from build123d import *

# Parameters (mm, degrees)
SKETCH1_W               = 37
SKETCH1_H               = 52
BOSS_EXTRUDE1_DEPTH     = 2
BOSS_EXTRUDE2_DEPTH     = 52
SKETCH3_W               = 10.2
SKETCH3_H               = 48.4
CUT_EXTRUDE1_DEPTH      = 11
CUT_EXTRUDE2_DEPTH      = 35.456494308
CUT_EXTRUDE2_DEPTH_BACK = 35.456494308


with BuildPart() as part:
    # Sketch1 → Boss-Extrude1 (new body)
    with BuildSketch(Plane.XY):
        Rectangle(SKETCH1_W, SKETCH1_H)
    extrude(amount=BOSS_EXTRUDE1_DEPTH)

    # Sketch2 → Boss-Extrude2 (add)
    with BuildSketch(Plane.XZ.offset(26)):
        with BuildLine():
            Line((-13.5, 13), (13.5, 13))
            ThreePointArc((13.5, 13), (17.035533906, 11.535533906), (18.5, 8))
            Line((18.5, 8), (18.5, 2))
            Line((18.5, 2), (-18.5, 2))
            Line((-18.5, 2), (-18.5, 8))
            ThreePointArc((-18.5, 8), (-17.035533906, 11.535533906), (-13.5, 13))
        make_face()
    extrude(amount=-BOSS_EXTRUDE2_DEPTH)

    # Sketch3 → Cut-Extrude1 (cut)
    with BuildSketch(Plane.XY.offset(13)):
        Rectangle(SKETCH3_W, SKETCH3_H)
        with Locations((11.4, 0)):
            Rectangle(SKETCH3_W, SKETCH3_H)
        with Locations((-11.4, 0)):
            Rectangle(SKETCH3_W, SKETCH3_H)
    extrude(amount=-CUT_EXTRUDE1_DEPTH, mode=Mode.SUBTRACT)

    # Sketch4 → Cut-Extrude2 (cut, two sides: drawn at the far end of the back side and taken through both)
    with BuildSketch(Plane(origin=(0, 0, 0), x_dir=(0, 0, -1), z_dir=(1, 0, 0)).offset(-CUT_EXTRUDE2_DEPTH_BACK)):
        Polygon((-18, -14.658032638), (-18, 14.658032638), (-8.2, 9), (-8.2, -9), align=None)
    extrude(amount=CUT_EXTRUDE2_DEPTH + CUT_EXTRUDE2_DEPTH_BACK, mode=Mode.SUBTRACT)


solid = part.part
The listing builds one solid part. Answer for the finished solid, in the listing's coordinates (mm). A direction names the side the tool comes from. Round coordinates to 2 decimals unless told otherwise and drop trailing zeros. Loops run counter-clockwise (first coordinate to the right, second up) from the corner with the lowest first, then second, coordinate; pieces in that order, holes last. Notation, with made-up numbers: M 67.25,63 L 91.25,63 A16 ccw 91.25,80 Z; hole C 6,-16.75 d3. An arc over 180 degrees is marked long. Return JSON: item names as keys, results as strings.
Q1. Find section C-C, the plane y = -16. Determine the outline of the cut face in (x, z), plus the area to 3 significant figures.
Results list:
{"outline": "M -18.5,0 L 18.5,0 L 18.5,8 A5 ccw 16.5,12 L 16.5,2 L 6.3,2 L 6.3,13 L 5.1,13 L 5.1,2 L -5.1,2 L -5.1,13 L -6.3,13 L -6.3,2 L -16.5,2 L -16.5,12 A5 ccw -18.5,8 Z", "area": "136 mm2"}
Q2. The mould has two halves that part along X. Classify faces 4 (the face through (-18, 0, 8.2)), 5 (the face through (11, -24.2, 8)), 6 (the face through (18.01, -11.92, 10.16)): released by +X, released by -X, zero draft, split by the parting line, or undercut.
Results list:
{"face 4": "zero draft", "face 5": "undercut", "face 6": "released by +X"}
Q3. Find the intervals of material crossed by line 1 along X through (y, z) = (20.5, 7); line 2 along Y through (x, z) = (-14, 5.75); line 3 along X through (y, z) = (12.5, 9.25), in increasing order. Write a range as from..to.
Results list:
{"line 1": "x = -18.5..-16.5, -6.3..-5.1, 5.1..6.3, 16.5..18.5", "line 2": "y = -26..-24.2, 24.2..26", "line 3": "x = -18.34..-16.5, -6.3..-5.1, 5.1..6.3, 16.5..18.34"}
Q4. Which of the six approach directions +Z, -Z, +X, -X, +Y, -Y give full straight-line access (tool end or side, diameter ignored) to faces 1 (the face through (18.5, 0, 4)), 2 (the face through (-16.5, 0, 7)), 3 (the face through (-17.29, 9.869, 9.704))?
Results list:
{"face 1": "+Z, -Z, +X, +Y, -Y", "face 2": "+Z", "face 3": "+Z, +X, -X"}
Q5. Find section B-B, the plane x = 0. Determine the outline of the cut face in (y, z).
Results list:
{"outline": "M -26,0 L 26,0 L 26,13 L 24.2,13 L 24.2,2 L -24.2,2 L -24.2,13 L -26,13 Z"}
Q6. Each of these flat-tipped pins is pushed along its axis until it touches: pin 1 Ø1.3 at (x, y) = (-6, 2.5) entering from +Z; pin 2 Ø1 at (x, y) = (11, 10.5) entering from +Z; pin 3 Ø2 at (y, z) = (6.5, 11) entering from -X. Where does it stop, or does it pass through?
Results list:
{"pin 1": "stops at z = 8.2", "pin 2": "stops at z = 2", "pin 3": "passes through"}
Q7. Find section A-A, the plane z = 6. Determine the outline of the cut face in (x, y), plus the area to 3 significant figures.
Results list:
{"outline": "M -18.5,-26 L 18.5,-26 L 18.5,26 L -18.5,26 Z; hole M -16.5,-24.2 L -6.3,-24.2 L -6.3,24.2 L -16.5,24.2 Z; hole M -5.1,-24.2 L 5.1,-24.2 L 5.1,24.2 L -5.1,24.2 Z; hole M 6.3,-24.2 L 16.5,-24.2 L 16.5,24.2 L 6.3,24.2 Z", "area": "443 mm2"}
